from build123d import *

# Parameters (mm, degrees)
SKETCH1_R           = 4.191
BOSS_EXTRUDE1_DEPTH = 1.3716
SKETCH2_R           = 3.175
BOSS_EXTRUDE2_DEPTH = 1.7272
SKETCH3_R           = 4.191
BOSS_EXTRUDE3_DEPTH = 1.3716
SKETCH4_R           = 1.5875
CUT_EXTRUDE1_DEPTH  = 5.4704
FILLET1_R           = 0.762


with BuildPart() as part:
    # Sketch1 → Boss-Extrude1 (new body)
    with BuildSketch(Plane(origin=(0, 0, 0), x_dir=(1, 0, 0), z_dir=(0, 1, 0))):
        Circle(SKETCH1_R)
    extrude(amount=BOSS_EXTRUDE1_DEPTH)

    # Sketch2 → Boss-Extrude2 (add)
    with BuildSketch(Plane(origin=(0, 1.3716, 0), x_dir=(1, 0, 0), z_dir=(0, 1, 0))):
        Circle(SKETCH2_R)
    extrude(amount=BOSS_EXTRUDE2_DEPTH)

    # Sketch3 → Boss-Extrude3 (add)
    with BuildSketch(Plane(origin=(0, 3.0988, 0), x_dir=(1, 0, 0), z_dir=(0, 1, 0))):
        Circle(SKETCH3_R)
    extrude(amount=BOSS_EXTRUDE3_DEPTH)

    # Sketch4 → Cut-Extrude1 (cut, through all)
    with BuildSketch(Plane(origin=(0, 4.4704, 0), x_dir=(1, 0, 0), z_dir=(0, 1, 0))):
        Circle(SKETCH4_R)
    extrude(amount=-CUT_EXTRUDE1_DEPTH, mode=Mode.SUBTRACT)

    # Fillet1
    fillet1_edges = [part.edges().sort_by_distance(p)[0] for p in [
        (-4.191, 4.4704, 0),
        (-4.191, 0, 0),
    ]]
    fillet(fillet1_edges, radius=FILLET1_R)


solid = part.part
Can you work these out from the model? Positions are in its coordinate system, mm. A direction names the side the tool comes from. Coordinates: 2 decimals unless noted, no trailing zeros. Loops run counter-clockwise (first coordinate to the right, second up) from the corner with the lowest first, then second, coordinate; pieces in that order, holes last. Notation, with made-up numbers: M -5,-27.75 L 26,-27.75 A24 ccw 26,11.25 Z; hole C -7,-29 d5. An arc over 180 degrees is marked long. Return JSON: item names as keys, results as strings. Group by question number.
Item 1: If I drill on L1, parallel to Y at x = 2.25, z = -2.5; L2, parallel to Z at x = 0, y = 2.65 (1 decimal), over which ranges is the centre line in solid material (lowest first)? Write a range as from..to.
Item 2: I'm going to push flat-ended pins straight in: pin 1 Ø3 at (x, z) = (0, 0) entering from +Y; pin 2 Ø2 at (x, y) = (-1.5, 1.5) entering from -Z. Where does each tip first touch, or does it pass through?
Item 3: Imagine slicing it at B-B (z = 0). Please give me the cut outline in (x, y) (1 decimal), and give its area (3 significant figures).
Item 4: Imagine slicing it at A-A (x = 0). Please give me the cut outline in (y, z) (1 decimal).
Item 5: Thinking about a two-plate mould opening in X: for faces 3 (the cylindrical face through (-0.34, 2.27, 1.55)), 4 (the flat face through (2, 1.372, -3)), 5 (the cylindrical face through (3.997, 3.399, -1.259)), which applies, released by +X, released by -X, zero draft, split by the parting line, or undercut?
Item 6: Imagine slicing it at D-D (y = 0.6). Please give me the cut outline in (x, z) (1 decimal), and give its area (3 significant figures).
Item 7: On a 3-axis mill with a long thin cutter (end or side, diameter ignored), from which of +Z, -Z, +X, -X, +Y, -Y can I reach the whole of each face in a straight line? I mean faces 1 (the flat face through (2, 3.099, -3)), 2 (the flat face through (1, 0, -2)). Say none if no direction works.
Verdict:
{
 "1": {"L1": "y = 0..1.37, 3.1..4.47", "L2": "z = -3.2..-1.6, 1.6..3.2"},
 "2": {"pin 1": "passes through", "pin 2": "stops at z = -4.16"},
 "3": {"outline": "M -4.2,0.8 A0.8 ccw -3.4,0 L -1.6,0 L -1.6,4.5 L -3.4,4.5 A0.8 ccw -4.2,3.7 L -4.2,3.1 L -3.2,3.1 L -3.2,1.4 L -4.2,1.4 Z; M 1.6,0 L 3.4,0 A0.8 ccw 4.2,0.8 L 4.2,1.4 L 3.2,1.4 L 3.2,3.1 L 4.2,3.1 L 4.2,3.7 A0.8 ccw 3.4,4.5 L 1.6,4.5 Z", "area": "19.3 mm^2"},
 "4": {"outline": "M 0,-3.4 A0.8 ccw 0.8,-4.2 L 1.4,-4.2 L 1.4,-3.2 L 3.1,-3.2 L 3.1,-4.2 L 3.7,-4.2 A0.8 ccw 4.5,-3.4 L 4.5,-1.6 L 0,-1.6 Z; M 0,1.6 L 4.5,1.6 L 4.5,3.4 A0.8 ccw 3.7,4.2 L 3.1,4.2 L 3.1,3.2 L 1.4,3.2 L 1.4,4.2 L 0.8,4.2 A0.8 ccw 0,3.4 Z"},
 "5": {"face 3": "undercut", "face 4": "zero draft", "face 5": "split by the parting line"},
 "6": {"outline": "C 0,0 d8.3; hole C 0,0 d3.2", "area": "46.8 mm^2"},
 "7": {"face 1": "none", "face 2": "+Z, -Z, +X, -X, -Y"}
}
